Model file for the job. Use its own axes, mm. Give positions to 0.01 mm unless a question says otherwise; leave off trailing zeros. Loops run counter-clockwise (first coordinate to the right, second up) from the corner with the lowest first, then second, coordinate; pieces in that order, holes last. Notation, with made-up numbers: (47, -16.75) - (70, -16.75) arc R17 ccw to (70, 9.25) - close; hole circle Ø2 at (-14, 36). An arc over 180 degrees is marked (long way). Use a Markdown table: item, result.
from build123d import *

# Parameters (mm, degrees)
F1_DEPTH = 5
F2_R     = 8
F3_DEPTH = 5.001


with BuildPart() as f1:
    # F0 (on Front) → F1 (new body)
    with BuildSketch(Plane.XZ):
        with BuildLine():
            Line((90, -123.110723), (17.628544, 11.946398))
            ThreePointArc((17.628544, 11.946398), (0, 22.5), (-17.628544, 11.946398))
            Line((-17.628544, 11.946398), (-90, -123.110723))
            ThreePointArc((-90, -123.110723), (0, -152.5), (90, -123.110723))
        make_face()
    extrude(amount=F1_DEPTH)

    # F2 (on face) → F3 (cut, through all)
    with BuildSketch(Plane.XZ.offset(5)):
        with Locations((0, 2.5)):
            Circle(F2_R)
    extrude(amount=-F3_DEPTH, mode=Mode.SUBTRACT)


solid = f1.part
(1) Mould opens along X. For faces 1 (the cylindrical face through (0.302, -2.465, 22.498)), 2 (the flat face through (-53.31, -2.46, -54.64)), 3 (the cylindrical face through (-1.73, -2.54, -5.31)), 4 (the flat face through (-1, 0, -83)) say: pulls with the +X half, pulls with the -X half, needs draft (parallel to the pull), parting line crosses it, or undercut.
Computed:
| item | result |
|---|---|
| face 1 | parting line crosses it |
| face 2 | pulls with the -X half |
| face 3 | undercut |
| face 4 | needs draft |
(2) Slice it at B-B, the plane y = -3.4. Write the cut outline in (x, z), plus the area to 3 significant figures.
Computed:
| item | result |
|---|---|
| outline | (-90, -123.11) arc R152.5 ccw to (90, -123.11) - (17.63, 11.95) arc R20 ccw to (-17.63, 11.95) - close; hole circle Ø16 at (0, 2.5) |
| area | 18,200 mm² |
(3) Slice it at D-D, the plane z = -43. Write the cut outline in (x, y), plus the area to 3 significant figures.
Computed:
| item | result |
|---|---|
| outline | (-47.07, -5) - (47.07, -5) - (47.07, 0) - (-47.07, 0) - close |
| area | 471 mm² |
(4) Slice it at C-C, the plane z = 2.5. Write the cut outline in (x, y).
Computed:
| item | result |
|---|---|
| outline | (-22.69, -5) - (-8, -5) - (-8, 0) - (-22.69, 0) - close; (8, -5) - (22.69, -5) - (22.69, 0) - (8, 0) - close |
(5) Slice it at A-A, the plane x = 0. Write the cut outline in (y, z).
Computed:
| item | result |
|---|---|
| outline | (-5, -152.5) - (0, -152.5) - (0, -5.5) - (-5, -5.5) - close; (-5, 10.5) - (0, 10.5) - (0, 22.5) - (-5, 22.5) - close |
(6) Drill centre lines: probe 1 along X at (y, z) = (-4.7, 9); probe 2 along X at (y, z) = (-4.3, 6); probe 3 along X at (y, z) = (-1.15, 12). Where is each one in solid material? Low to high. Write a range as [from, to].
Computed:
| item | result |
|---|---|
| probe 1 | [-19.21, -4.66], [4.66, 19.21] |
| probe 2 | [-20.81, -7.19], [7.19, 20.81] |
| probe 3 | [-17.6, 17.6] |
(7) Pin check, flat tips, straight feed: P1, Ø1.5, axis at y = -2.5, z = -10, coming from the +X side; P2, Ø2, axis at y = -4, z = -104.5, coming from the +X side; P3, Ø1, axis at x = -32, y = -1, coming from the -Z side. Stop position of each tip, or through.
Computed:
| item | result |
|---|---|
| P1 | x = 29.79 |
| P2 | x = 80.56 |
| P3 | z = -149.21 |
